Could you check a few things on this model? Use its own coordinates, in mm. Face numbers are marked on the shaded views. Coordinates: 2 decimals unless noted, no trailing zeros. Order: outer loops, then holes, each group sorted by start corner. A loop starts at its lowest first (then second) coordinate and runs counter-clockwise, first axis right, second up. Notation, with made-up numbers: (2, 43.25) -> (51, 43.25) arc R22 ccw to (51, 62.25) -> close; hole circle Ø2 at (59, 63). An arc over 180 degrees is marked (long way). Put each result on its own line as item: value. Start each with the question number.
Q1. If we section it at A-A (z = 0): Please give me the cut outline in (x, y) (3 decimals).
Q2. Will these pins go through, and if not, where does the flat tip stop? pin 1 (0.8 mm diameter, centred on x = 26.5, z = -0.5, fed in from +Y); pin 2 (5 mm diameter, centred on x = 55, y = 0.5, fed in from +Z).
Q3. We'd pull the mould along Y, two halves only. Please class the marked faces 1 and 2: +Y half, -Y half, draft (parallel to the pull), parting line (faces both ways), or undercut.
Q4. Please list where these lines run through material, in increasing order: line 1 along Z through (x, y) = (16.5, 0) (3 decimals); line 2 along Y through (x, z) = (41.5, 4.5); line 3 along Z through (x, y) = (57, 6.25).
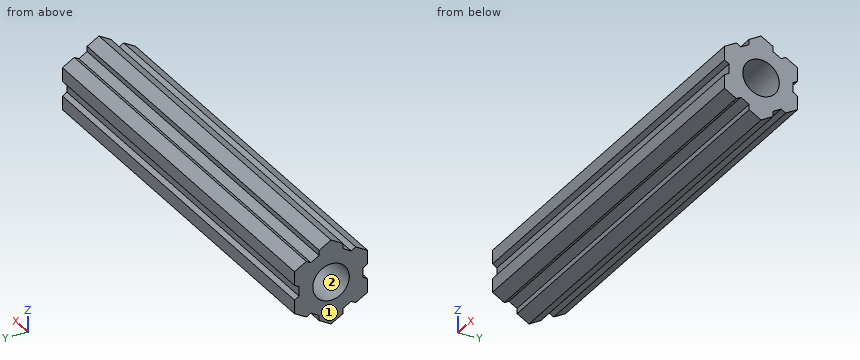
Autodesk Inventor part; units mm, degrees
ref_plane "YZ Plane" through (0, 0, 0) normal (1, 0, 0) x (0, 1, 0)
ref_plane "XZ Plane" through (0, 0, 0) normal (0, 1, 0) x (-1, 0, 0)
ref_plane "XY Plane" through (0, 0, 0) normal (0, 0, 1) x (1, 0, 0)
sketch "Sketch1" plane through (0, 0, 0) normal (1, 0, 0) x (0, 1, 0)
  line L0 (6.35, 3.6662) -> (6.35, -3.6662) construction
  line L1 (6.35, -3.6662) -> (0, -7.3323) construction
  line L2 (0, -7.3323) -> (-6.35, -3.6662) construction
  line L3 (-6.35, -3.6662) -> (-6.35, 3.6662) construction
  line L4 (-6.35, 3.6662) -> (0, 7.3323) construction
  line L5 (0, 7.3323) -> (6.35, 3.6662) construction
  line L6 (5.5563, -3.2079) -> (5.5563, 3.2079) construction
  line L7 (5.5563, 3.2079) -> (0, 6.4158) construction
  line L8 (0, 6.4158) -> (-5.5563, 3.2079) construction
  line L9 (-5.5563, 3.2079) -> (-5.5563, -3.2079) construction
  line L10 (-5.5563, -3.2079) -> (0, -6.4158) construction
  line L11 (0, -6.4158) -> (5.5563, -3.2079) construction
  line L12 (6.35, 3.6662) -> (6.35, 1.2849)
  line L13 (6.35, 3.6662) -> (4.2878, 4.8568)
  line L14 (6.35, -3.6662) -> (6.35, -1.2849)
  line L15 (6.35, -3.6662) -> (4.2878, -4.8568)
  line L16 (0, -7.3323) -> (2.0622, -6.1417)
  line L17 (0, -7.3323) -> (-2.0622, -6.1417)
  line L18 (-6.35, -3.6662) -> (-4.2878, -4.8568)
  line L19 (-6.35, -3.6662) -> (-6.35, -1.2849)
  line L20 (-6.35, 3.6662) -> (-6.35, 1.2849)
  line L21 (-6.35, 3.6662) -> (-4.2878, 4.8568)
  line L22 (0, 7.3323) -> (2.0622, 6.1417)
  line L23 (0, 7.3323) -> (-2.0622, 6.1417)
  line L24 (6.35, 1.2849) -> (5.5563, 0.8267)
  line L25 (6.35, 1.2849) -> (7.2665, 1.2849) construction
  line L26 (6.35, -1.2849) -> (5.5563, -0.8267)
  line L27 (6.35, -1.2849) -> (7.2665, -1.2849) construction
  line L28 (5.5563, -0.8267) -> (5.5563, 0.8267)
  line L29 (4.2878, -4.8568) -> (3.494, -4.3985)
  line L30 (4.2878, -4.8568) -> (5.2043, -4.8568) construction
  line L31 (2.0622, -6.1417) -> (2.0622, -5.2252)
  line L32 (2.0622, -6.1417) -> (2.9788, -6.1417) construction
  line L33 (-2.0622, -6.1417) -> (-2.0622, -5.2252)
  line L34 (-2.0622, -6.1417) -> (-1.1457, -6.1417) construction
  line L35 (3.494, -4.3985) -> (2.0622, -5.2252)
  line L36 (-4.2878, -4.8568) -> (-3.494, -4.3985)
  line L37 (-4.2878, -4.8568) -> (-3.3712, -4.8568) construction
  line L38 (-3.494, -4.3985) -> (-2.0622, -5.2252)
  line L39 (-6.35, -1.2849) -> (-5.5563, -0.8267)
  line L40 (-6.35, -1.2849) -> (-5.4335, -1.2849) construction
  line L41 (-6.35, 1.2849) -> (-5.5563, 0.8267)
  line L42 (-6.35, 1.2849) -> (-5.4335, 1.2849) construction
  line L43 (-5.5563, 0.8267) -> (-5.5563, -0.8267)
  line L44 (-4.2878, 4.8568) -> (-3.494, 4.3985)
  line L45 (-4.2878, 4.8568) -> (-3.3712, 4.8568) construction
  line L46 (-2.0622, 6.1417) -> (-2.0622, 5.2252)
  line L47 (-2.0622, 6.1417) -> (-1.1457, 6.1417) construction
  line L48 (-2.0622, 5.2252) -> (-3.494, 4.3985)
  line L49 (2.0622, 6.1417) -> (2.0622, 5.2252)
  line L50 (2.0622, 6.1417) -> (2.9788, 6.1417) construction
  line L51 (4.2878, 4.8568) -> (3.494, 4.3985)
  line L52 (4.2878, 4.8568) -> (5.2043, 4.8568) construction
  line L53 (3.494, 4.3985) -> (2.0622, 5.2252)
  circle A0 centre (0, 0) radius 3.175
  dimension "d0" = 12.7
  dimension "d1" = 12.7
  dimension "d2" = 12.7
  dimension "d3" = 120
  dimension "d4" = 120
  dimension "d5" = 6.35
  dimension "d6" = 6.35
  dimension "d7" = 6.35
  dimension "d11" = 0.7937
  dimension "d12" = 2.3813
  dimension "d13" = 2.3813
  dimension "d14" = 2.3813
  dimension "d15" = 2.3813
  dimension "d16" = 2.3813
  dimension "d17" = 2.3813
  dimension "d18" = 2.3813
  dimension "d19" = 2.3813
  dimension "d20" = 2.3813
  dimension "d21" = 2.3813
  dimension "d22" = 2.3813
  dimension "d23" = 2.3813
  dimension "d24" = 150
  dimension "d25" = 150
  dimension "d26" = 150
  dimension "d27" = 90
  dimension "d28" = 90
  dimension "d29" = 30
  dimension "d30" = 30
  dimension "d31" = 30
  dimension "d32" = 30
  dimension "d33" = 90
  dimension "d34" = 90
  dimension "d35" = 150
  dimension "d36" = 6.35
extrude "Extrusion1" add sketch "Sketch1" along normal blind 69.85
properties part number "churro" material "Aluminum 6061"
The answers:
1. outline: (0, -5.556) -> (69.85, -5.556) -> (69.85, -3.175) -> (0, -3.175) -> close; (0, 3.175) -> (69.85, 3.175) -> (69.85, 5.556) -> (0, 5.556) -> close
2. pin 1: y = 5.68
2. pin 2: z = 7.33
3. face 1: draft
3. face 2: undercut
4. line 1: -7.332 to -3.175, 3.175 to 7.332
4. line 2: -4.91 to -3.67, -3.32 to 3.32, 3.67 to 4.91
4. line 3: -3.72 to -1.23, 1.23 to 3.72
